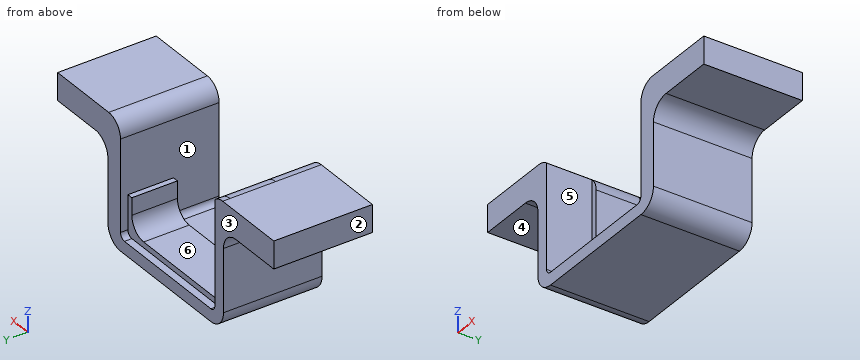
from build123d import *

# Parameters (mm, degrees)
BOSS_EXTRUDE1_DEPTH = 4
BOSS_EXTRUDE2_DEPTH = 0.65
BOSS_EXTRUDE3_START = 4
BOSS_EXTRUDE3_DEPTH = 4


with BuildPart() as part:
    # Sketch1 → Boss-Extrude1 (new body)
    with BuildSketch(Plane(origin=(0, 0, 0), x_dir=(1, 0, 0), z_dir=(0, 1, 0))):
        with BuildLine():
            Line((-5.5, -3.002039615), (-5.5, 4))
            ThreePointArc((-5.5, 4), (-5.353553391, 4.353553391), (-5, 4.5))
            Line((-5, 4.5), (4, 4.5))
            ThreePointArc((4, 4.5), (5.060660172, 4.060660172), (5.5, 3))
            Line((5.5, 3), (5.5, 1.5))
            Line((5.5, 1.5), (6, 1.5))
            Line((6, 1.5), (6, -3.5))
            ThreePointArc((6, -3.5), (6.439339828, -4.560660172), (7.5, -5))
            Line((7.5, -5), (14, -5))
            Line((14, -5), (14, -2.6))
            Line((14, -2.6), (9.2, -2.6))
            ThreePointArc((9.2, -2.6), (8.06862915, -2.13137085), (7.6, -1))
            Line((7.6, -1), (7.6, 4.5))
            ThreePointArc((7.6, 4.5), (7.13137085, 5.63137085), (6, 6.1))
            Line((6, 6.1), (-5.5, 6.1))
            ThreePointArc((-5.5, 6.1), (-6.63137085, 5.63137085), (-7.1, 4.5))
            Line((-7.1, 4.5), (-7.1, -1))
            ThreePointArc((-7.1, -1), (-7.56862915, -2.13137085), (-8.7, -2.6))
            Line((-8.7, -2.6), (-13.5, -2.6))
            Line((-13.5, -2.6), (-13.5, -5))
            Line((-13.5, -5), (-7, -5))
            ThreePointArc((-7, -5), (-5.939339828, -4.560660172), (-5.5, -3.5))
            Line((-5.5, -3.5), (-5.5, -3.002039615))
        make_face()
    extrude(amount=BOSS_EXTRUDE1_DEPTH)

    # Sketch2 → Boss-Extrude2 (add)
    with BuildSketch(Plane(origin=(0, 4, 0), x_dir=(1, 0, 0), z_dir=(0, 1, 0))):
        with BuildLine():
            Line((-13.5, -5), (-7, -5))
            ThreePointArc((-7, -5), (-6.457416135, -4.898428671), (-5.988313555, -4.607470332))
            ThreePointArc((-5.988313555, -4.607470332), (-5.997069803, -4.554051932), (-6, -4.5))
            Line((-6, -4.5), (-6, 4.5))
            ThreePointArc((-6, 4.5), (-5.853553391, 4.853553391), (-5.5, 5))
            Line((-5.5, 5), (5.5, 5))
            ThreePointArc((5.5, 5), (5.853553391, 4.853553391), (6, 4.5))
            Line((6, 4.5), (6, -3.5))
            ThreePointArc((6, -3.5), (6.439339828, -4.560660172), (7.5, -5))
            Line((7.5, -5), (14, -5))
            Line((14, -5), (14, -2.6))
            Line((14, -2.6), (9.2, -2.6))
            ThreePointArc((9.2, -2.6), (8.06862915, -2.13137085), (7.6, -1))
            Line((7.6, -1), (7.6, 4.5))
            ThreePointArc((7.6, 4.5), (7.13137085, 5.63137085), (6, 6.1))
            Line((6, 6.1), (-5.5, 6.1))
            ThreePointArc((-5.5, 6.1), (-6.63137085, 5.63137085), (-7.1, 4.5))
            Line((-7.1, 4.5), (-7.1, -1))
            ThreePointArc((-7.1, -1), (-7.56862915, -2.13137085), (-8.7, -2.6))
            Line((-8.7, -2.6), (-13.5, -2.6))
            Line((-13.5, -2.6), (-13.5, -5))
        make_face()
    extrude(amount=BOSS_EXTRUDE2_DEPTH)

    # Sketch3 → Boss-Extrude3 (add)
    with BuildSketch(Plane.XZ.offset(BOSS_EXTRUDE3_START)):
        with BuildLine():
            Line((7.6, -4.5), (7.6, 1))
            ThreePointArc((7.6, 1), (8.06862915, 2.13137085), (9.2, 2.6))
            Line((9.2, 2.6), (14, 2.6))
            Line((14, 2.6), (14, 5))
            Line((14, 5), (7.5, 5))
            ThreePointArc((7.5, 5), (6.439339828, 4.560660172), (6, 3.5))
            Line((6, 3.5), (6, 2.6))
            Line((6, 2.6), (6, -1.5))
            Line((6, -1.5), (6, -4.5))
            ThreePointArc((6, -4.5), (5.853553391, -4.853553391), (5.5, -5))
            Line((5.5, -5), (-5.5, -5))
            ThreePointArc((-5.5, -5), (-5.853553391, -4.853553391), (-6, -4.5))
            Line((-6, -4.5), (-6, 2.6))
            Line((-6, 2.6), (-6, 4.5))
            Line((-6, 4.5), (-6, 4.618033989))
            ThreePointArc((-6, 4.618033989), (-6.464766865, 4.901258538), (-7, 5))
            Line((-7, 5), (-13.5, 5))
            Line((-13.5, 5), (-13.5, 2.6))
            Line((-13.5, 2.6), (-8.7, 2.6))
            ThreePointArc((-8.7, 2.6), (-7.56862915, 2.13137085), (-7.1, 1))
            Line((-7.1, 1), (-7.1, -4.5))
            ThreePointArc((-7.1, -4.5), (-6.63137085, -5.63137085), (-5.5, -6.1))
            Line((-5.5, -6.1), (6, -6.1))
            ThreePointArc((6, -6.1), (7.13137085, -5.63137085), (7.6, -4.5))
        make_face()
    extrude(amount=-BOSS_EXTRUDE3_DEPTH)


solid = part.part
Geometry check sheet. Reference: the model listing, model coordinates, mm. Face numbers are marked on the shaded views. A direction names the side the tool comes from. Round coordinates to 2 decimals unless told otherwise and drop trailing zeros. Write each loop counter-clockwise with the first axis right and the second up, starting at its lowest first coordinate (ties: lowest second). Pieces come first, ordered by that corner, then holes.
Item 1: Section check C-C (y = 2.5). Record the boundary of the cut face in (x, z).
Determined:
outline: (-13.5, 2.6) - (-8.7, 2.6) arc R1.6 cw to (-7.1, 1) - (-7.1, -4.5) arc R1.6 ccw to (-5.5, -6.1) - (6, -6.1) arc R1.6 ccw to (7.6, -4.5) - (7.6, 1) arc R1.6 cw to (9.2, 2.6) - (14, 2.6) - (14, 5) - (7.5, 5) arc R1.5 ccw to (6, 3.5) - (6, -1.5) - (5.5, -1.5) - (5.5, -3) arc R1.5 cw to (4, -4.5) - (-5, -4.5) arc R0.5 cw to (-5.5, -4) - (-5.5, 3.5) arc R1.5 ccw to (-7, 5) - (-13.5, 5) - close
Item 2: Access from +Z, -Z, +X, -X, +Y, -Y to the whole of each face (thin tool, end or side, straight path). Record for the marked faces 4, 5 and 6.
Determined:
face 4: -Z, -X, +Y, -Y
face 5: +Z, -Y
face 6: +Z, +Y, -Y
Item 3: Section check A-A (z = 0.5). Record the boundary of the cut face in (x, y).
Determined:
outline: (-7.1, -4) - (-6, -4) - (-6, 0) - (-5.5, 0) - (-5.5, 4) - (-6, 4) - (-6, 4.65) - (-7.1, 4.65) - close; (6, -4) - (7.6, -4) - (7.6, 4.65) - (6, 4.65) - close
Item 4: Go/stop test with flat-tipped pins: pin 1 Ø0.5 at (x, y) = (-2, 4) entering from +Z; pin 2 Ø4 at (y, z) = (0, -2) entering from -X; pin 3 Ø4 at (y, z) = (1.5, -0.5) entering from -X. Record where each tip stops, or that it passes through.
Determined:
pin 1: stops at z = -4.5
pin 2: stops at x = -7.1
pin 3: stops at x = -7.18
Item 5: Mould release check, pull along X, two halves, no side actions. Record for the marked faces 1, 2 and 3: +X half, -X half, draft (parallel to the pull), parting line (faces both ways), or undercut.
Determined:
face 1: undercut
face 2: -X half
face 3: draft
Item 6: Section check D-D (z = 3). Record the boundary of the cut face in (x, y).
Determined:
outline: (-13.5, -4) - (-6, -4) - (-6, 0) - (-5.5, 0) - (-5.5, 4) - (-6, 4) - (-6, 4.65) - (-13.5, 4.65) - close; (6, -4) - (14, -4) - (14, 4.65) - (6, 4.65) - close
Item 7: Material ranges on line 1 along X through (y, z) = (2.25, -1); line 2 along X through (y, z) = (1.5, -3); line 3 along Z through (x, y) = (-3.25, -1.25), recorded low to high.
Determined:
line 1: x = -7.1 to -5.5, 6 to 7.6
line 2: x = -7.1 to -5.5, 5.5 to 7.6
line 3: z = -6.1 to -5
Item 8: Section check B-B (x = -2). Record the boundary of the cut face in (y, z).
Determined:
outline: (-4, -6.1) - (4.65, -6.1) - (4.65, -5) - (4, -5) - (4, -4.5) - (0, -4.5) - (0, -5) - (-4, -5) - close
